Part print with two shaded views. Sizes in mm from the minimum x, y, z corner. A direction names the side the tool comes from. Give positions to 0.01 mm unless a question says otherwise; leave off trailing zeros. Write each loop counter-clockwise with the first axis right and the second up, starting at its lowest first coordinate (ties: lowest second). Pieces come first, ordered by that corner, then holes. Notation, with made-up numbers: M -28.5,-29 L -24.5,-29 A19 ccw -24.5,-5 Z; hole C 64.5,13.25 d3. An arc over 180 degrees is marked long. One line per item, written item: value. Start each with the question number.
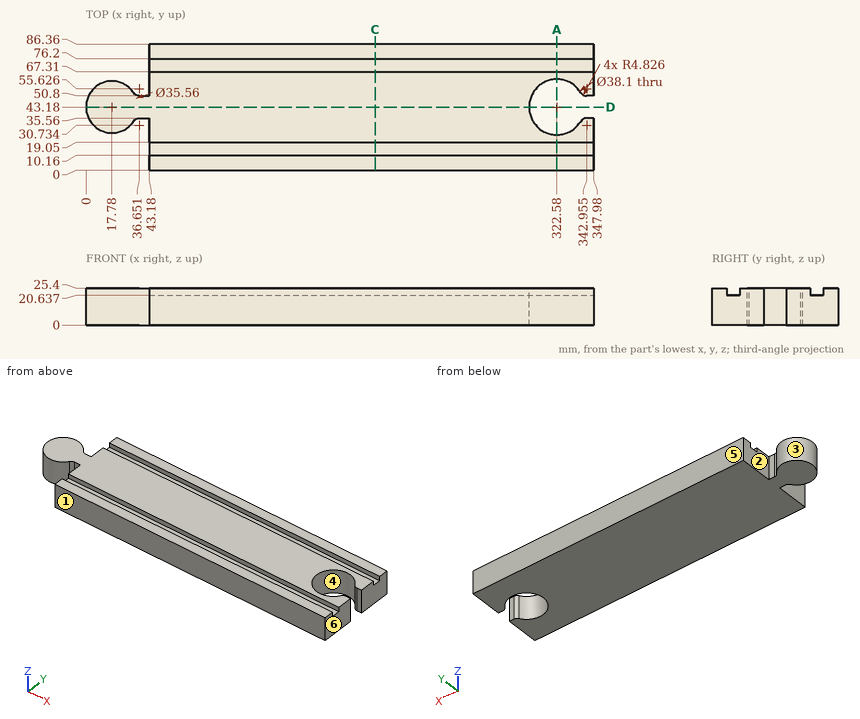
1) Tool access for the marked faces 1 and 2: list every direction of +Z, -Z, +X, -X, +Y, -Y with a clear straight run to the whole face (end or side of a thin tool).
2) Drop flat-ended pins along their axis: P1, Ø5, axis at x = 40, z = 17, coming from the -Y side; P2, Ø4.5, axis at x = 220, y = 15.5, coming from the +Z side; P3, Ø3.5, axis at x = 40.5, z = 18.5, coming from the +Y side; P4, Ø2, axis at x = 42, y = 24, coming from the +Z side. Give the stop position or say it passes through.
3) Mould opens along X. For the marked faces 3, 4, 5 and 6 say: released by +X, released by -X, zero draft, split by the parting line, or undercut.
4) Band-saw the part on D-D (y = 43.18). List the corners of the cut face in (x, z).
5) Band-saw the part on C-C (x = 198). List the corners of the cut face in (y, z).
6) Probe line 1 along Y through (x, z) = (322.58, 9.5); line 2 along X through (y, z) = (56, 6.75); line 3 along X through (y, z) = (24, 17.25). List the from-to ranges inside material, lowest first. Write a range as from..to.
7) Band-saw the part on A-A (x = 322.58). List the corners of the cut face in (y, z), then the cut area to 3 significant figures.
Model answer:
1. face 1: +Z, -Z, +X, -X, -Y
1. face 2: +Z, -Z, +Y
2. P1: stops at y = 35.56
2. P2: stops at z = 20.64
2. P3: stops at y = 50.8
2. P4: passes through
3. face 3: undercut
3. face 4: undercut
3. face 5: zero draft
3. face 6: released by +X
4. outline: M 0,0 L 303.53,0 L 303.53,25.4 L 0,25.4 Z
5. outline: M 0,0 L 86.36,0 L 86.36,25.4 L 76.2,25.4 L 76.2,20.64 L 67.31,20.64 L 67.31,25.4 L 19.05,25.4 L 19.05,20.64 L 10.16,20.64 L 10.16,25.4 L 0,25.4 Z
6. line 1: y = 0..24.13, 62.23..86.36
6. line 2: x = 5.46..30.1, 43.18..308.49, 336.67..347.98
6. line 3: x = 43.18..347.98
7. outline: M 0,0 L 24.13,0 L 24.13,25.4 L 19.05,25.4 L 19.05,20.64 L 10.16,20.64 L 10.16,25.4 L 0,25.4 Z; M 62.23,0 L 86.36,0 L 86.36,25.4 L 76.2,25.4 L 76.2,20.64 L 67.31,20.64 L 67.31,25.4 L 62.23,25.4 Z
7. area: 1,140 mm²
